Verification items for the finished model (mm, model axes). A direction names the side the tool comes from. Coordinates: 2 decimals unless noted, no trailing zeros. Loops run counter-clockwise (first coordinate to the right, second up) from the corner with the lowest first, then second, coordinate; pieces in that order, holes last. Notation, with made-up numbers: (18, 6) - (58, 6) arc R15 cw to (58, 12) - close; hole circle Ø2 at (-29.5, 54). An arc over 180 degrees is marked (long way). One line per item, written item: value. Start each with the question number.
(1) Section check A-A (x = 0). Record the boundary of the cut face in (y, z).
(2) Thickness scan on probe 1 along Y at (x, z) = (0, 4.85); probe 2 along X at (y, z) = (54, 1.5); probe 3 along Y at (x, z) = (5, 5). Record the ranges inside material, lowest first. Write a range as [from, to].
(3) Section check D-D (x = -5). Record the boundary of the cut face in (y, z).
(4) Set-up check for faces 1 (the face through (9.31, 59.426, 4.53)), 2 (the face through (0, 2, 3.1)): record each of +Z, -Z, +X, -X, +Y, -Y from which the full face is reachable in a straight line by a thin tool's end or side.
(5) Section check C-C (z = -0.5). Record the boundary of the cut face in (x, y), plus the area to 3 significant figures.
(6) Gauge pin test, flat ends, axial feed: P1, Ø4.5, axis at x = -9.52, y = 57.79, coming from the -Z side; P2, Ø3, axis at x = 9.52, y = 57.79, coming from the -Z side; P3, Ø4.5, axis at x = 0, y = 0, coming from the +Z side. Record the tip position at first contact, or that the pin passes through.
(7) Draft check along Y on faces 3 (the face through (14.196, 60.275, 0.514)), 4 (the face through (16.66, -60.42, 2.06)), 5 (the face through (-18.079, 0, 2)). Enter one of: +Y half, -Y half, draft (parallel to the pull), parting line (faces both ways), or undercut.
(8) Section check B-B (y = 0). Record the boundary of the cut face in (x, z), plus the area to 3 significant figures.
```python
from build123d import *

# Parameters (mm, degrees)
F1_START      = 3.1
F0_W          = 32
F0_H          = 122
F0_R          = 1.65
F0_R_2        = 1.25
F0_R_3        = 12.75
F1_DEPTH      = 2.9
F2_START      = 3
F0_R_4        = 2
F0_R_5        = 1
F2_DEPTH      = 2
F3_DEPTH      = 25
F3_DEPTH_BACK = 39.8
F0_W_2        = 36.2426135689
F0_H_2        = 125.9943731129
F4_DEPTH      = 2
F4_DEPTH_BACK = 6
F5_R          = 6
F6_R          = 5


# Not quite as in the source:
# - a feature names something its author has since deleted; it is built from what else it names


with BuildPart() as f1:
    # F0 (on Top) → F1 (new body)
    with BuildSketch(Plane.XY.offset(F1_START)):
        with Locations((0, 0.9860133167)):
            Rectangle(F0_W, F0_H)
        with Locations((-9.525, -57.4329458177)):
            Circle(F0_R, mode=Mode.SUBTRACT)
        with Locations((-9.525, -30.4671674967)):
            Circle(F0_R_2, mode=Mode.SUBTRACT)
        with Locations((0, -44.4789328166)):
            Circle(F0_R_3, mode=Mode.SUBTRACT)
        with Locations((-9.525, 0)):
            Circle(F0_R_2, mode=Mode.SUBTRACT)
        with Locations((0, -15.4157546586)):
            Circle(F0_R_3, mode=Mode.SUBTRACT)
        Circle(F0_R, mode=Mode.SUBTRACT)
        with Locations((9.525, -57.4329458177)):
            Circle(F0_R, mode=Mode.SUBTRACT)
        with Locations((9.525, -30.4671674967)):
            Circle(F0_R_2, mode=Mode.SUBTRACT)
        with Locations((9.525, 0)):
            Circle(F0_R_2, mode=Mode.SUBTRACT)
        with Locations((-9.525, 29.1974432766)):
            Circle(F0_R_2, mode=Mode.SUBTRACT)
        with Locations((0, 15.3948861798)):
            Circle(F0_R_3, mode=Mode.SUBTRACT)
        with Locations((-9.525, 57.7905103564)):
            Circle(F0_R, mode=Mode.SUBTRACT)
        with Locations((0, 44.3624239764)):
            Circle(F0_R_3, mode=Mode.SUBTRACT)
        with Locations((9.525, 29.1974432766)):
            Circle(F0_R_2, mode=Mode.SUBTRACT)
        with Locations((9.525, 57.7905103564)):
            Circle(F0_R, mode=Mode.SUBTRACT)
        with Locations((9.525, 0)):
            Circle(F0_R_2)
        with Locations((-9.525, 0)):
            Circle(F0_R_2)
        with Locations((9.525, 29.1974432766)):
            Circle(F0_R_2)
        with Locations((-9.525, 29.1974432766)):
            Circle(F0_R_2)
        with Locations((9.525, -30.4671674967)):
            Circle(F0_R_2)
        with Locations((-9.525, -30.4671674967)):
            Circle(F0_R_2)
        with Locations((9.525, -57.4329458177)):
            Circle(F0_R)
        with Locations((-9.525, -57.4329458177)):
            Circle(F0_R)
        Circle(F0_R)
        with Locations((9.525, 57.7905103564)):
            Circle(F0_R)
        with Locations((-9.525, 57.7905103564)):
            Circle(F0_R)
    extrude(amount=F1_DEPTH)

    # F0 (on Top) → F2 (cut)
    with BuildSketch(Plane.XY.offset(F2_START)):
        with Locations((0, 44.3624239764)):
            Circle(F0_R_3)
        with Locations((-9.525, 44.3624239764)):
            Circle(F0_R_4, mode=Mode.SUBTRACT)
        with Locations((9.525, 44.3624239764)):
            Circle(F0_R_4, mode=Mode.SUBTRACT)
        with Locations((0, 15.3948861798)):
            Circle(F0_R_3)
        with Locations((-9.525, 15.3948861798)):
            Circle(F0_R_4, mode=Mode.SUBTRACT)
        with Locations((9.525, 15.3948861798)):
            Circle(F0_R_4, mode=Mode.SUBTRACT)
        with Locations((0, -15.4157546586)):
            Circle(F0_R_3)
        with Locations((-9.525, -15.4157546586)):
            Circle(F0_R_4, mode=Mode.SUBTRACT)
        with Locations((9.525, -15.4157546586)):
            Circle(F0_R_4, mode=Mode.SUBTRACT)
        with Locations((0, -44.4789328166)):
            Circle(F0_R_3)
        with Locations((-9.525, -44.4789328166)):
            Circle(F0_R_4, mode=Mode.SUBTRACT)
        with Locations((9.525, -44.4789328166)):
            Circle(F0_R_4, mode=Mode.SUBTRACT)
        with Locations((9.525, 44.3624239764)):
            Circle(F0_R_4)
        with Locations((9.525, 44.3624239764)):
            Circle(F0_R_5, mode=Mode.SUBTRACT)
        with Locations((-9.525, 44.3624239764)):
            Circle(F0_R_4)
        with Locations((-9.525, 44.3624239764)):
            Circle(F0_R_5, mode=Mode.SUBTRACT)
        with Locations((9.525, 15.3948861798)):
            Circle(F0_R_4)
        with Locations((9.525, 15.3948861798)):
            Circle(F0_R_5, mode=Mode.SUBTRACT)
        with Locations((-9.525, 15.3948861798)):
            Circle(F0_R_4)
        with Locations((-9.525, 15.3948861798)):
            Circle(F0_R_5, mode=Mode.SUBTRACT)
        with Locations((9.525, -15.4157546586)):
            Circle(F0_R_4)
        with Locations((9.525, -15.4157546586)):
            Circle(F0_R_5, mode=Mode.SUBTRACT)
        with Locations((-9.525, -15.4157546586)):
            Circle(F0_R_4)
        with Locations((-9.525, -15.4157546586)):
            Circle(F0_R_5, mode=Mode.SUBTRACT)
        with Locations((9.525, -44.4789328166)):
            Circle(F0_R_4)
        with Locations((9.525, -44.4789328166)):
            Circle(F0_R_5, mode=Mode.SUBTRACT)
        with Locations((-9.525, -44.4789328166)):
            Circle(F0_R_4)
        with Locations((-9.525, -44.4789328166)):
            Circle(F0_R_5, mode=Mode.SUBTRACT)
        with Locations((9.525, 44.3624239764)):
            Circle(F0_R_5)
        with Locations((-9.525, 44.3624239764)):
            Circle(F0_R_5)
        with Locations((9.525, 15.3948861798)):
            Circle(F0_R_5)
        with Locations((-9.525, 15.3948861798)):
            Circle(F0_R_5)
        with Locations((9.525, -15.4157546586)):
            Circle(F0_R_5)
        with Locations((-9.525, -15.4157546586)):
            Circle(F0_R_5)
        with Locations((9.525, -44.4789328166)):
            Circle(F0_R_5)
        with Locations((-9.525, -44.4789328166)):
            Circle(F0_R_5)
    extrude(amount=F2_DEPTH, mode=Mode.SUBTRACT)

    # F0 (on Top) → F3 (cut, two sides)
    with BuildSketch(Plane.XY) as f3_sk:
        with Locations((9.525, -57.4329458177)):
            Circle(F0_R)
        Circle(F0_R)
        with Locations((-9.525, -57.4329458177)):
            Circle(F0_R)
        with Locations((-9.525, 57.7905103564)):
            Circle(F0_R)
        with Locations((9.525, 57.7905103564)):
            Circle(F0_R)
    extrude(amount=-F3_DEPTH, mode=Mode.SUBTRACT)
    extrude(f3_sk.sketch, amount=F3_DEPTH_BACK, mode=Mode.SUBTRACT)

    # F0 (on Top) → F4 (join, two sides)
    with BuildSketch(Plane.XY) as f4_sk:
        with Locations((0.0427393243, 1.1539515108)):
            Rectangle(F0_W_2, F0_H_2)
        with Locations((0, 0.9860133167)):
            Rectangle(F0_W, F0_H, mode=Mode.SUBTRACT)
    extrude(amount=-F4_DEPTH)
    extrude(f4_sk.sketch, amount=F4_DEPTH_BACK)

    # F5
    f5_edges = [f1.edges().sort_by_distance(p)[0] for p in [
        (-16, -60.013987, 0.55),
        (16, -60.013987, 0.55),
        (-16, 61.986013, 0.55),
        (16, 61.986013, 0.55),
    ]]
    fillet(f5_edges, radius=F5_R)

    # F6
    f6_edges = [f1.edges().sort_by_distance(p)[0] for p in [
        (18.164046, 64.151138, 2),
        (-18.078567, 64.151138, 2),
        (-18.078567, -61.843235, 2),
        (18.164046, -61.843235, 2),
    ]]
    fillet(f6_edges, radius=F6_R)


solid = f1.part
```
Responses:
1. outline: (-61.84, -2) - (-60.01, -2) - (-60.01, 3.1) - (-57.23, 3.1) - (-57.23, 6) - (-61.84, 6) - close; (-31.73, 3.1) - (-28.17, 3.1) - (-28.17, 6) - (-31.73, 6) - close; (-2.67, 3.1) - (-1.65, 3.1) - (-1.65, 6) - (-2.67, 6) - close; (1.65, 3.1) - (2.64, 3.1) - (2.64, 6) - (1.65, 6) - close; (28.14, 3.1) - (31.61, 3.1) - (31.61, 6) - (28.14, 6) - close; (57.11, 3.1) - (61.99, 3.1) - (61.99, -2) - (64.15, -2) - (64.15, 6) - (57.11, 6) - close
2. probe 1: y = [-61.84, -57.23], [-31.73, -28.17], [-2.67, -1.65], [1.65, 2.64], [28.14, 31.61], [57.11, 64.15]
2. probe 2: x = [-18.08, -16], [16, 18.16]
2. probe 3: y = [-61.84, -56.21], [-32.75, -27.14], [-3.69, 3.67], [27.12, 32.63], [56.09, 64.15]
3. outline: (-61.84, -2) - (-60.01, -2) - (-60.01, 3.1) - (-56.21, 3.1) - (-56.21, 6) - (-61.84, 6) - close; (-32.75, 3.1) - (-27.14, 3.1) - (-27.14, 6) - (-32.75, 6) - close; (-3.69, 3.1) - (3.67, 3.1) - (3.67, 6) - (-3.69, 6) - close; (27.12, 3.1) - (32.63, 3.1) - (32.63, 6) - (27.12, 6) - close; (56.09, 3.1) - (61.99, 3.1) - (61.99, -2) - (64.15, -2) - (64.15, 6) - (56.09, 6) - close
4. face 1: +Z, -Z
4. face 2: -Z
5. outline: (-18.08, -56.84) arc R5 ccw to (-13.08, -61.84) - (13.16, -61.84) arc R5 ccw to (18.16, -56.84) - (18.16, 59.15) arc R5 ccw to (13.16, 64.15) - (-13.08, 64.15) arc R5 ccw to (-18.08, 59.15) - close; hole (-16, -54.01) arc R6 ccw to (-10, -60.01) - (10, -60.01) arc R6 ccw to (16, -54.01) - (16, 55.99) arc R6 ccw to (10, 61.99) - (-10, 61.99) arc R6 ccw to (-16, 55.99) - close
5. area: 672 mm²
6. P1: stops at z = 3.1
6. P2: passes through
6. P3: stops at z = 6
7. face 3: undercut
7. face 4: -Y half
7. face 5: draft
8. outline: (-18.08, -2) - (-16, -2) - (-16, 3.1) - (-1.65, 3.1) - (-1.65, 6) - (-18.08, 6) - close; (1.65, 3.1) - (16, 3.1) - (16, -2) - (18.16, -2) - (18.16, 6) - (1.65, 6) - close
8. area: 117 mm²
